CAD build for the part. Positions are in the model's coordinates, mm. Coordinates: 2 decimals unless noted, no trailing zeros. Loops run counter-clockwise (first coordinate to the right, second up) from the corner with the lowest first, then second, coordinate; pieces in that order, holes last.
1) Saw through at D-D, the plane x = 4. Write the cut outline in (y, z) (3 decimals).
2) Wall check: line 1 along X through (y, z) = (4.5, -1); line 2 along X through (y, z) = (0.5, -2.5); line 3 along Z through (x, y) = (9, 2.5) (3 decimals). Give the ranges that are in metal, low to high.
3) Saw through at C-C, the plane x = -2. Write the cut outline in (y, z) (3 decimals).
4) Saw through at A-A, the plane z = -2.75. Write the cut outline in (x, y).
5) Saw through at B-B, the plane y = 2.75. Write the cut outline in (x, z) (3 decimals), and give its area (3 significant figures).
```python
from build123d import *

# Parameters (mm, degrees)
SKETCH1_W           = 50.8
SKETCH1_H           = 11.43
BOSS_EXTRUDE1_DEPTH = 6.35
CUT_EXTRUDE1_DEPTH  = 7.35


with BuildPart() as part:
    # Sketch1 → Boss-Extrude1 (new body)
    with BuildSketch(Plane(origin=(0, 0, 0), x_dir=(1, 0, 0), z_dir=(0, 1, 0))):
        Rectangle(SKETCH1_W, SKETCH1_H)
    extrude(amount=BOSS_EXTRUDE1_DEPTH)

    # Sketch2 → Cut-Extrude1 (cut, through all)
    with BuildSketch(Plane(origin=(0, 6.35, 0), x_dir=(1, 0, 0), z_dir=(0, 1, 0))):
        with BuildLine():
            Line((-9.525, 5.715), (9.525, 5.715))
            ThreePointArc((9.525, 5.715), (0, 0), (-9.525, 5.715))
        make_face()
    extrude(amount=-CUT_EXTRUDE1_DEPTH, mode=Mode.SUBTRACT)


solid = part.part
```
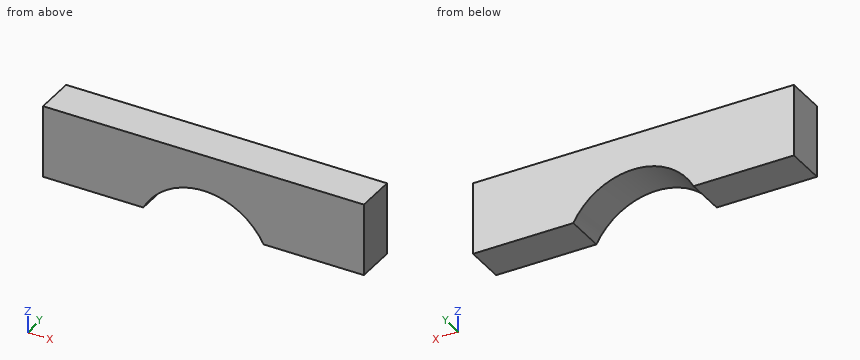
Data:
1. outline: (0, -0.768) - (6.35, -0.768) - (6.35, 5.715) - (0, 5.715) - close
2. line 1: x = -25.4 to -4.54, 4.54 to 25.4
2. line 2: x = -25.4 to -6.91, 6.91 to 25.4
2. line 3: z = -4.834 to 5.715
3. outline: (0, -0.187) - (6.35, -0.187) - (6.35, 5.715) - (0, 5.715) - close
4. outline: (-25.4, 0) - (-7.2, 0) - (-7.2, 6.35) - (-25.4, 6.35) - close; (7.2, 0) - (25.4, 0) - (25.4, 6.35) - (7.2, 6.35) - close
5. outline: (-25.4, -5.715) - (-9.525, -5.715) arc R10.795 cw to (9.525, -5.715) - (25.4, -5.715) - (25.4, 5.715) - (-25.4, 5.715) - close
5. area: 503 mm2
